Autodesk Inventor part; units mm, degrees
ref_plane "YZ Plane" through (0, 0, 0) normal (1, 0, 0) x (0, 1, 0)
ref_plane "XZ Plane" through (0, 0, 0) normal (0, 1, 0) x (-1, 0, 0)
ref_plane "XY Plane" through (0, 0, 0) normal (0, 0, 1) x (1, 0, 0)
sketch "Sketch1" plane through (0, 0, 0) normal (0, 0, 1) x (1, 0, 0)
  line L0 (-609.6, -63.5) -> (609.6, -63.5)
  line L1 (609.6, 63.5) -> (-609.6, 63.5)
  line L2 (-609.6, -63.5) -> (609.6, 63.5) construction
  line L3 (609.6, -63.5) -> (-609.6, 63.5) construction
  line L4 (-609.6, 63.5) -> (-609.6, -12.7)
  line L5 (-609.6, -12.7) -> (-933.45, -12.7)
  line L6 (-933.45, -12.7) -> (-933.45, -63.5)
  line L7 (-933.45, -63.5) -> (-609.6, -63.5)
  line L8 (609.6, -63.5) -> (933.45, -63.5)
  line L9 (933.45, -63.5) -> (933.45, -12.7)
  line L10 (933.45, -12.7) -> (609.6, -12.7)
  line L11 (609.6, -12.7) -> (609.6, 63.5)
  line L12 (0, 88.9) -> (0, -88.9)
  point P0 (0, 0)
  dimension "d0" = 127
  dimension "d1" = 1219.2
  dimension "d2" = 323.85
  dimension "d3" = 50.8
extrude "Extrusion1" add sketch "Sketch1" along normal blind 19.05
fillet "Fillet1" radius 19.05 4 edges at (-609.6, -12.7, 9.525) (-609.6, 63.5, 9.525) (609.6, 63.5, 9.525) (609.6, -12.7, 9.525)
ref_plane "Work Plane2" through (-933.45, -38.1, 19.05) normal (0, 1, 0) x (1, 0, 0)
ref_plane "Work Plane3" through (-628.65, -12.7, 0) normal (-1, 0, 0) x (0, 0, 1)
ref_plane "Work Plane4" through (628.65, -12.7, 0) normal (1, 0, 0) x (0, 0, -1)
equation "\"d2\" = ELength"
equation "\"d3\" = EHeight"
equation "\"d4\" = Thickness"
equation "\"Thickness\" = 19.05"
equation "\"EHeight\" = 50.8"
equation "\"ELength\" = 323.85"
properties part number "Frame"
For this review, take the finished solid that the model builds, in its own axes (mm). Give positions to 0.01 mm unless a question says otherwise; leave off trailing zeros. Order: outer loops, then holes, each group sorted by start corner. A loop starts at its lowest first (then second) coordinate and runs counter-clockwise, first axis right, second up.
1) Take a section at C-C (y = 24). Give the boundary of the cut face in (x, z).
2) Wall thickness on line 1 (X direction, y = 19.5, z = 4.25); line 2 (Y direction, x = 799.5, z = 4.25); line 3 (X direction, y = -8, z = 6.75): over which ranges is each line inside the solid? List them lowest first.
3) Insertion check: pin 1 (6 mm diameter, centred on y = 47.5, z = 9.5, fed in from +X); pin 2 (5.5 mm diameter, centred on x = 785, z = 8.5, fed in from +Y); pin 3 (6 mm diameter, centred on x = -592.5, y = 20.5, fed in from -Z). Each pin has a flat end and moves straight along its axis. Give the tip position at first contact, or say it passes through.
4) Take a section at A-A (z = 9.5). Give the boundary of the cut face in (x, y).
5) Take a section at B-B (x = 739). Give the boundary of the cut face in (y, z).
Derived:
1. outline: (-609.6, 0) - (609.6, 0) - (609.6, 19.05) - (-609.6, 19.05) - close
2. line 1: x = -609.6 to 609.6
2. line 2: y = -63.5 to -12.7
2. line 3: x = -616.12 to 616.12
3. pin 1: stops at x = 609.6
3. pin 2: stops at y = -12.7
3. pin 3: stops at z = 0
4. outline: (-933.45, -63.5) - (933.45, -63.5) - (933.45, -12.7) - (628.65, -12.7) arc R19.05 cw to (609.6, 6.35) - (609.6, 44.45) arc R19.05 ccw to (590.55, 63.5) - (-590.55, 63.5) arc R19.05 ccw to (-609.6, 44.45) - (-609.6, 6.35) arc R19.05 cw to (-628.65, -12.7) - (-933.45, -12.7) - close
5. outline: (-63.5, 0) - (-12.7, 0) - (-12.7, 19.05) - (-63.5, 19.05) - close
